Geometry: see drawing. Coordinates: mm, zero at the bounding-box minimum. Round coordinates to 2 decimals unless told otherwise and drop trailing zeros. Order: outer loops, then holes, each group sorted by start corner. A loop starts at its lowest first (then second) coordinate and runs counter-clockwise, first axis right, second up. Notation, with made-up numbers: (-32, 30.5) -> (2, 30.5) arc R20 ccw to (2, 38.5) -> close; hole circle Ø6 at (-19, 35.5). An arc over 180 degrees is marked (long way). Use a Markdown table: item, result.
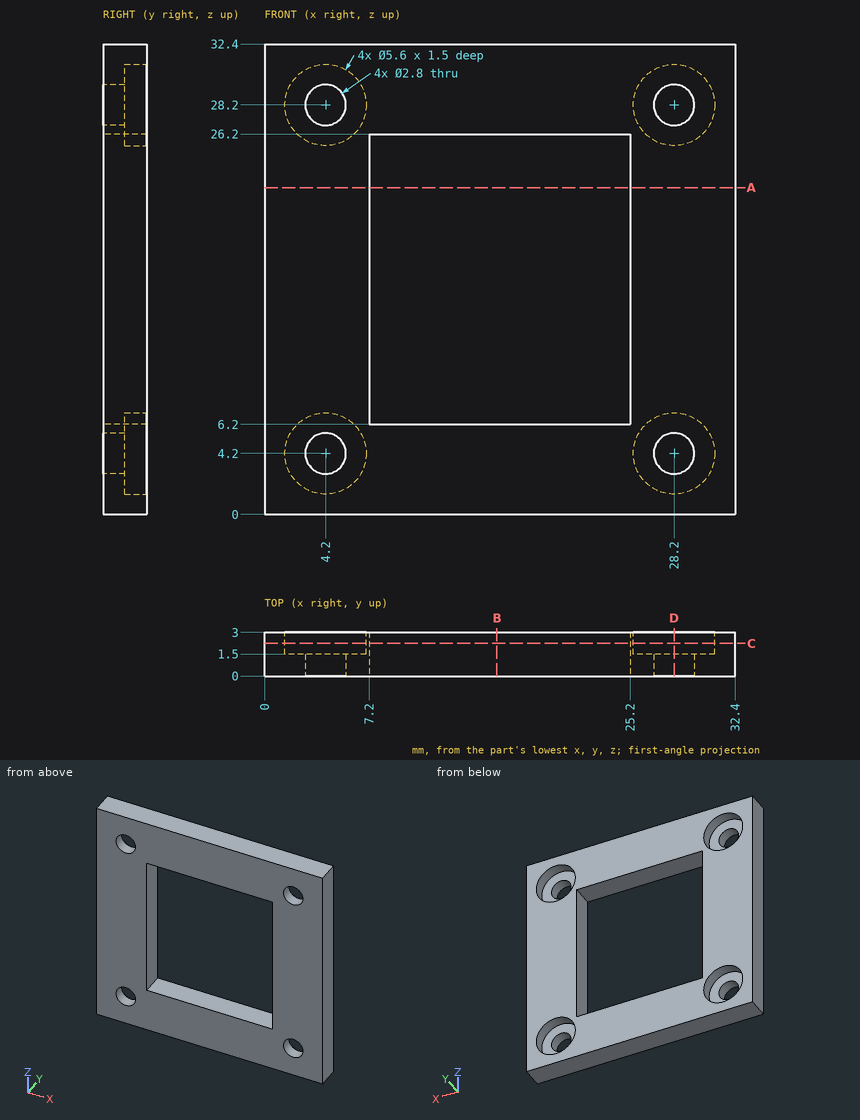
1) Contact query for flat-ended pins moving along their axis: P1, Ø4.5, axis at x = 4.2, z = 4.2, coming from the +Y side; P2, Ø2, axis at x = 4.2, z = 28.2, coming from the +Y side. Output: stop coordinate, or through.
Answer key:
| item | result |
|---|---|
| P1 | stops at y = 1.5 |
| P2 | passes through |
2) Cut plane C-C on y = 2.25. Return loops of the section in (x, z).
Answer key:
| item | result |
|---|---|
| outline | (0, 0) -> (32.4, 0) -> (32.4, 32.4) -> (0, 32.4) -> close; hole circle Ø5.6 at (4.2, 4.2); hole circle Ø5.6 at (4.2, 28.2); hole (7.2, 6.2) -> (25.2, 6.2) -> (25.2, 26.2) -> (7.2, 26.2) -> close; hole circle Ø5.6 at (28.2, 4.2); hole circle Ø5.6 at (28.2, 28.2) |
3) Ray query, probe 1 along Z at (x, y) = (28.2, 1.9); probe 2 along X at (y, z) = (0.35, 4.2). Return the intervals inside material, ascending.
Answer key:
| item | result |
|---|---|
| probe 1 | z = 0 to 1.4, 7 to 25.4, 31 to 32.4 |
| probe 2 | x = 0 to 2.8, 5.6 to 26.8, 29.6 to 32.4 |
4) Cut plane A-A on z = 22.5. Return loops of the section in (x, y), and give its area (3 significant figures).
Answer key:
| item | result |
|---|---|
| outline | (0, 0) -> (7.2, 0) -> (7.2, 3) -> (0, 3) -> close; (25.2, 0) -> (32.4, 0) -> (32.4, 3) -> (25.2, 3) -> close |
| area | 43.2 mm^2 |
5) Cut plane D-D on x = 28.2. Return loops of the section in (y, z).
Answer key:
| item | result |
|---|---|
| outline | (0, 0) -> (3, 0) -> (3, 1.4) -> (1.5, 1.4) -> (1.5, 2.8) -> (0, 2.8) -> close; (0, 5.6) -> (1.5, 5.6) -> (1.5, 7) -> (3, 7) -> (3, 25.4) -> (1.5, 25.4) -> (1.5, 26.8) -> (0, 26.8) -> close; (0, 29.6) -> (1.5, 29.6) -> (1.5, 31) -> (3, 31) -> (3, 32.4) -> (0, 32.4) -> close |
6) Cut plane B-B on x = 16. Return loops of the section in (y, z).
Answer key:
| item | result |
|---|---|
| outline | (0, 0) -> (3, 0) -> (3, 6.2) -> (0, 6.2) -> close; (0, 26.2) -> (3, 26.2) -> (3, 32.4) -> (0, 32.4) -> close |
